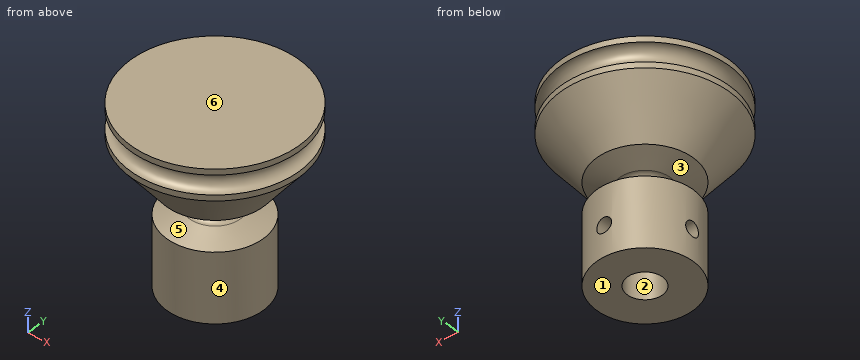
```python
from build123d import *

# Parameters (mm, degrees)
F0_R     = 0.975
F2_DEPTH = 6.6
F3_R     = 0.975
F4_DEPTH = 6.6


with BuildPart() as f1:
    # F0 (on Front) → F1 (revolve)
    with BuildSketch(Plane.XZ):
        with BuildLine():
            Line((-6.3, 0), (-2.3, 0))
            Line((-2.3, 0), (-2.3, 8))
            Line((-2.3, 8), (0, 8))
            Line((0, 8), (0, 23))
            Line((0, 23), (-11, 23))
            Line((-11, 23), (-11, 22.25))
            ThreePointArc((-11, 22.25), (-9.75, 21), (-11, 19.75))
            Line((-11, 19.75), (-11, 19))
            Line((-11, 19), (-6.3, 13))
            Line((-6.3, 13), (-3.3, 12))
            ThreePointArc((-3.3, 12), (-2.3, 11), (-3.3, 10))
            Line((-3.3, 10), (-6.3, 9))
            Line((-6.3, 9), (-6.3, 0))
        make_face()
    revolve(axis=Axis((0, 0, 15.5), (0, 0, 1)))

    # F0 (on Front) → F2 (cut)
    with BuildSketch(Plane.XZ):
        with Locations((0, 4)):
            Circle(F0_R)
    extrude(amount=-F2_DEPTH, mode=Mode.SUBTRACT)

    # F3 (on Right) → F4 (cut)
    with BuildSketch(Plane.YZ):
        with Locations((0, 4)):
            Circle(F3_R)
    extrude(amount=-F4_DEPTH, mode=Mode.SUBTRACT)


solid = f1.part
```
Work out the finished part from the listing and answer in its coordinate system (mm). Face numbers are marked on the shaded views. A direction names the side the tool comes from. Round coordinates to 2 decimals unless told otherwise and drop trailing zeros. Order: outer loops, then holes, each group sorted by start corner. A loop starts at its lowest first (then second) coordinate and runs counter-clockwise, first axis right, second up.
Q1. A cutting plane is placed at B-B, the plane y = 0. Determine the outline of the cut face in (x, z) (3 decimals).
Solution:
outline: (-11, 19) - (-6.3, 13) - (-3.3, 12) arc R1 cw to (-3.3, 10) - (-6.3, 9) - (-6.3, 4.975) - (-2.3, 4.975) - (-2.3, 8) - (2.3, 8) - (2.3, 0) - (6.3, 0) - (6.3, 9) - (3.3, 10) arc R1 cw to (3.3, 12) - (6.3, 13) - (11, 19) - (11, 19.75) arc R1.25 cw to (11, 22.25) - (11, 23) - (-11, 23) - (-11, 22.25) arc R1.25 cw to (-11, 19.75) - close; (-6.3, 0) - (-2.3, 0) - (-2.3, 3.025) - (-6.3, 3.025) - close
Q2. A cutting plane is placed at A-A, the plane x = 0. Determine the outline of the cut face in (y, z) (3 decimals), then the cut area to 3 significant figures.
Solution:
outline: (-11, 19) - (-6.3, 13) - (-3.3, 12) arc R1 cw to (-3.3, 10) - (-6.3, 9) - (-6.3, 0) - (-2.3, 0) - (-2.3, 8) - (2.3, 8) - (2.3, 4.975) - (6.3, 4.975) - (6.3, 9) - (3.3, 10) arc R1 cw to (3.3, 12) - (6.3, 13) - (11, 19) - (11, 19.75) arc R1.25 cw to (11, 22.25) - (11, 23) - (-11, 23) - (-11, 22.25) arc R1.25 cw to (-11, 19.75) - close; (2.3, 0) - (6.3, 0) - (6.3, 3.025) - (2.3, 3.025) - close
area: 285 mm2
Q3. A cutting plane is placed at C-C, the plane z = 5.75. Determine the outline of the cut face in (x, y).
Solution:
outline: circle Ø12.6 at (0, 0); hole circle Ø4.6 at (0, 0)
Q4. Find the intervals of material crossed by line 1 along Z through (x, y) = (-3.1, 0) (3 decimals); line 2 along Y through (x, z) = (0, 2.25); line 3 along Z through (x, y) = (0, 3.5) (3 decimals), in increasing order.
Solution:
line 1: z = 0 to 3.025, 4.975 to 10.02, 11.98 to 23
line 2: y = -6.3 to -2.3, 2.3 to 6.3
line 3: z = 0 to 3.025, 4.975 to 9.933, 12.067 to 23
Q5. A tool of negligible diameter and unlimited length cuts with its end or side. For the marked faces 4, 5 and 6, from which of +Z, -Z, +X, -X, +Y, -Y can it reach the whole face along a straight path? Write none if from no direction.
Solution:
face 4: -Z
face 5: none
face 6: +Z, +X, -X, +Y, -Y
Q6. The mould has two halves that part along X. Classify the marked faces 1, 2 and 3: pulls with the +X half, pulls with the -X half, needs draft (parallel to the pull), parting line crosses it, or undercut.
Solution:
face 1: needs draft
face 2: undercut
face 3: parting line crosses it
Q7. A cutting plane is placed at D-D, the plane z = 14.5. Determine the outline of the cut face in (x, y) (3 decimals).
Solution:
outline: circle Ø14.95 at (0, 0)
Q8. Given pin 1 Ø12 at (y, z) = (8, 19.5) entering from +X; pin 2 Ø2.5 at (y, z) = (0, 4) entering from -X; pin 3 Ø8 at (x, z) = (-7.5, 18) entering from -Y, each flat-ended and moving along its own axis, determine where each tip first touches the part or whether it passes through.
Solution:
pin 1: stops at x = 10.82
pin 2: stops at x = -6.3
pin 3: stops at y = -10.38
